The model under review builds one solid part; all positions refer to its coordinate system, in mm. A direction names the side the tool comes from. Coordinates: 2 decimals unless noted, no trailing zeros. Write each loop counter-clockwise with the first axis right and the second up, starting at its lowest first coordinate (ties: lowest second). Pieces come first, ordered by that corner, then holes. Notation, with made-up numbers: (-38.5, 43.5) - (20.5, 43.5) arc R6 cw to (20.5, 50.5) - close; hole circle Ø10 at (21, 13). An arc over 180 degrees is marked (long way). Put each result on its own line as item: value.
from build123d import *

# Parameters (mm, degrees)
EXTRUDE_1_DEPTH = 12
EXTRUDE_2_DEPTH = 1


with BuildPart() as part:
    # 草图1 → 凸台-拉伸1 (new body)
    with BuildSketch(Plane(origin=(0, 0, 0), x_dir=(1, 0, 0), z_dir=(0, 1, 0))):
        Polygon((0, 0), (0, 21), (10, 21), (10, 6), (25, 6), (25, 0), align=None)
        Polygon((1, 20), (9, 20), (9, 5), (24, 5), (24, 1), (1, 1), align=None, mode=Mode.SUBTRACT)
    extrude(amount=EXTRUDE_1_DEPTH)

    # 草图3 → 凸台-拉伸2 (add)
    with BuildSketch(Plane.XZ):
        Polygon((10, -21), (0, -21), (0, 0), (25, 0), (25, -6), (10, -6), align=None)
    extrude(amount=EXTRUDE_2_DEPTH)


solid = part.part
1. To check wall thickness, follow probe 1 along X at (y, z) = (6, -13); probe 2 along Z at (x, y) = (16, 3); probe 3 along X at (y, z) = (4.75, -1.5). State the ranges of each line that lie inside material, in increasing order.
Determined:
probe 1: x = 0 to 1, 9 to 10
probe 2: z = -6 to -5, -1 to 0
probe 3: x = 0 to 1, 24 to 25
2. The part is to be moulded in two halves that separate along Z. For faces 4 (the flat face through (9, 6, -13)), 5 (the flat face through (12, 6, 0)), 6 (the flat face through (0, 6, -11)), say which applies: +Z half, -Z half, draft (parallel to the pull), parting line (faces both ways), or undercut.
Determined:
face 4: undercut
face 5: +Z half
face 6: draft
3. Consider section C-C on y = 8.75. State the section outline as (x, z) points, plus the area to 3 significant figures.
Determined:
outline: (0, -21) - (10, -21) - (10, -6) - (25, -6) - (25, 0) - (0, 0) - close; hole (1, -20) - (9, -20) - (9, -5) - (24, -5) - (24, -1) - (1, -1) - close
area: 88.0 mm^2
4. Consider section A-A on x = 9.5. State the section outline as (y, z) points, plus the area to 3 significant figures.
Determined:
outline: (-1, -21) - (12, -21) - (12, -5) - (0, -5) - (0, -1) - (12, -1) - (12, 0) - (-1, 0) - close
area: 225 mm^2
5. For pin 1 Ø6.5 at (y, z) = (2.5, -15) entering from +X; pin 2 Ø6 at (x, y) = (17, 6) entering from -Z, all flat-tipped, find the tip position at first contact; note any pin that passes through.
Determined:
pin 1: stops at x = 10
pin 2: stops at z = -6
6. Consider section B-B on z = -11. State the section outline as (x, y) points.
Determined:
outline: (0, -1) - (10, -1) - (10, 12) - (9, 12) - (9, 0) - (1, 0) - (1, 12) - (0, 12) - close
7. Machinability: for faces 1 (the flat face through (9.8, 12, -8.2)), 2 (the flat face through (1, 6, -10)), 3 (the flat face through (18, 6, -6)), which of the approach directions +Z, -Z, +X, -X, +Y, -Y give a long, thin tool a straight path to every point of the face, cutting with its end or side? Answer none if there is none.
Determined:
face 1: +Z, -Z, +X, -X, +Y
face 2: +Y
face 3: -Z, +X, +Y, -Y
